CAD build for the part. Positions are in the model's coordinates, mm. A direction names the side the tool comes from. Coordinates: 2 decimals unless noted, no trailing zeros. Loops run counter-clockwise (first coordinate to the right, second up) from the corner with the lowest first, then second, coordinate; pieces in that order, holes last. Notation, with made-up numbers: (83.5, 46) -> (91.5, 46) arc R31 cw to (91.5, 78) -> close; hole circle Ø6 at (41.25, 65). An arc over 180 degrees is marked (long way). Answer as a JSON object with one key per item and string values. Group by question number.
from build123d import *

# Parameters (mm, degrees)
ESBO_O3_W                  = 45
ESBO_O3_H                  = 1.9
CORTE_EXTRUS_O1_DEPTH      = 34.063063068
CORTE_EXTRUS_O1_DEPTH_BACK = 34.063063068
ESBO_O4_R                  = 2.75
ESBO_O5_R                  = 2.75
CORTE_EXTRUS_O2_DEPTH      = 34.971447122
FILETE1_R                  = 4


with BuildPart() as part:
    # Varredura2: sweep along a path in Esboço1
    with BuildLine(Plane.XY) as varredura2_path:
        Line((-16.822580645, 6.096774194), (-16.822580645, -14.903225806))
        Line((-16.822580645, -14.903225806), (4.177419355, -14.903225806))
    # Esboço3 → Varredura2 (sweep)
    with BuildSketch(Plane(origin=(4.177419355, 0, 0), x_dir=(0, 0, -1), z_dir=(1, 0, 0))):
        with Locations((0, -13.953225806)):
            Rectangle(ESBO_O3_W, ESBO_O3_H)
    sweep(path=varredura2_path.line, transition=Transition.RIGHT)

    # Esboço4 → Corte-extrusão1 (cut, two sides: drawn at the far end of the back side and taken through both)
    with BuildSketch(Plane(origin=(-14.922580645, 0, 0), x_dir=(0, 0, -1), z_dir=(1, 0, 0)).offset(-CORTE_EXTRUS_O1_DEPTH_BACK)):
        with Locations((0, 2.096774194)):
            Circle(ESBO_O4_R)
        Polygon((0, 6.096774194), (-3, 6.096774194), (-11.25, -13.003225806), (-24.249816644, -13.003225806), (-24.249816644, 8.86202898), (24.249816644, 8.86202898), (24.249816644, -13.003225806), (11.25, -13.003225806), (3, 6.096774194), align=None)
    extrude(amount=CORTE_EXTRUS_O1_DEPTH + CORTE_EXTRUS_O1_DEPTH_BACK, mode=Mode.SUBTRACT)

    # Esboço5 → Corte-extrusão2 (cut, symmetric)
    with BuildSketch(Plane(origin=(0, -13.003225806, 0), x_dir=(1, 0, 0), z_dir=(0, 1, 0))):
        with Locations(Location((0.177419355, -18.5, 0), (0, 0, 270))):
            Circle(ESBO_O5_R)
        Polygon((-14.922580645, -11.25), (-18.889664127, -11.25), (-18.889664127, -25.413435485), (7.454666431, -25.413435485), (7.454666431, -2.187603421), (4.177419355, -2.187603421), (4.177419355, -22.5), (-2.92481363, -22.5), align=None)
    corte_extrus_o2 = extrude(amount=CORTE_EXTRUS_O2_DEPTH, both=True, mode=Mode.SUBTRACT)

    # Espelhar1: Corte-extrusão2 across plane
    add(corte_extrus_o2.mirror(Plane.XY), mode=Mode.SUBTRACT)

    # Filete1
    filete1_edges = [part.edges().sort_by_distance(p)[0] for p in [
        (4.177419355, -13.953225806, -22.5),
        (4.177419355, -13.953225806, 22.5),
        (-2.92481363, -13.953225806, -22.5),
        (-15.872580645, 6.096774194, -3),
        (-15.872580645, 6.096774194, 3),
        (-2.92481363, -13.953225806, 22.5),
    ]]
    fillet(filete1_edges, radius=FILETE1_R)


solid = part.part
Item 1: Pull direction X, two halves, no side cores. Call faces 3 (the cylindrical face through (0.298, -13.94, 15.753)), 4 (the flat face through (-14.923, -6, 0)), 5 (the flat face through (-5, -13.003, 0)), 6 (the cylindrical face through (0.298, -13.94, -15.753)): +X half, -X half, draft (parallel to the pull), parting line (faces both ways), or undercut.
Item 2: Flat gauge pins, fed straight in: P1, Ø8, axis at y = -6.5, z = -15, coming from the +X side; P2, Ø6.5, axis at y = 2.1, z = 0, coming from the +X side; P3, Ø8, axis at y = 0, z = -9, coming from the -X side; P4, Ø1.5, axis at x = -16, y = -14, coming from the -Z side. Where does each tip first touch, or does it go through?
Item 3: 3-axis set-ups, long thin cutter, end or side, ignore diameter. For faces 1 (the flat face through (-16, -14, 11.25)), 2 (the cylindrical face through (2.975, -13.94, -21.359)): which of +Z, -Z, +X, -X, +Y, -Y reach the whole face in a straight line?
Item 4: Band-saw the part on A-A, the plane x = 0.75. List the corners of the cut face in (y, z), and give its area (3 significant figures).
Item 5: Band-saw the part on D-D, the plane x = -2. List the corners of the cut face in (y, z).
Item 6: Drill centre lines: L1, parallel to Y at x = -16.1, z = 0; L2, parallel to X at y = -2.5, z = -1.5; L3, parallel to Y at x = 1.5, z = -3. Where is each one in solid material? Low to high.
Item 7: Band-saw the part on C-C, the plane y = -4.25. List the corners of the cut face in (x, z).
Item 8: Band-saw the part on B-B, the plane z = 18. List the corners of the cut face in (x, y).
Reply:
{
 "1": {"face 3": "undercut", "face 4": "+X half", "face 5": "draft", "face 6": "undercut"},
 "2": {"P1": "through", "P2": "x = -14.92", "P3": "x = -16.82", "P4": "z = -11.25"},
 "3": {"face 1": "+Z, -X, +Y, -Y", "face 2": "-Z, +X, +Y, -Y"},
 "4": {"outline": "(-14.9, -22.46) -> (-13, -22.46) -> (-13, -21.19) -> (-14.9, -21.19) -> close; (-14.9, -15.81) -> (-13, -15.81) -> (-13, 15.81) -> (-14.9, 15.81) -> close; (-14.9, 21.19) -> (-13, 21.19) -> (-13, 22.46) -> (-14.9, 22.46) -> close", "area": "64.9 mm²"},
 "5": {"outline": "(-14.9, -22.45) -> (-13, -22.45) -> (-13, -20.18) -> (-14.9, -20.18) -> close; (-14.9, -16.82) -> (-13, -16.82) -> (-13, 16.82) -> (-14.9, 16.82) -> close; (-14.9, 20.18) -> (-13, 20.18) -> (-13, 22.45) -> (-14.9, 22.45) -> close"},
 "6": {"L1": "-14.9 to -0.65, 4.85 to 6.1", "L2": "-16.82 to -14.92", "L3": "-14.9 to -13"},
 "7": {"outline": "(-16.82, -7.47) -> (-14.92, -7.47) -> (-14.92, 7.47) -> (-16.82, 7.47) -> close"},
 "8": {"outline": "(-7.72, -14.9) -> (-2.53, -14.9) -> (-2.53, -13) -> (-7.72, -13) -> close; (2.88, -14.9) -> (4.18, -14.9) -> (4.18, -13) -> (2.88, -13) -> close"}
}
